Could you check a few things on this model? Use its own coordinates, in mm. A direction names the side the tool comes from. Round coordinates to 2 decimals unless told otherwise and drop trailing zeros. Loops run counter-clockwise (first coordinate to the right, second up) from the corner with the lowest first, then second, coordinate; pieces in that order, holes last. Notation, with made-up numbers: M -32.5,67 L -27.5,67 A12 cw -27.5,72 Z; hole C 50.5,84.5 d9. An arc over 180 degrees is marked long. One line per item, written item: value. Start each with the question number.
Q1. I'm going to push flat-ended pins straight in: pin 1 Ø1.4 at (x, y) = (77, 71) entering from +Z; pin 2 Ø5 at (x, y) = (55.12, 44.7) entering from +Z; pin 3 Ø2 at (y, z) = (64.5, 21) entering from -X. Where does each tip first touch, or does it pass through?
Q2. Imagine slicing it at A-A (y = 31.75). Please give me the cut outline in (x, z) (3 decimals).
Q3. Please list where these lines run through material, in increasing order: line 1 along Y through (x, z) = (5.08, 25.5) (3 decimals); line 2 along X through (y, z) = (78.5, 40); line 3 along Y through (x, z) = (7, 38.5).
Q4. Imagine slicing it at C-C (x = 67). Please give me the cut outline in (y, z), then the cut area to 3 significant figures.
Q5. Which directions (+Z, -Z, +X, -X, +Y, -Y) give clear straight access to the entire face, cutting with the end or side of a thin tool? Please do faces 1 (the face through (139.6, 93.2, 23.93)), 2 (the face through (14.41, 74.89, 10.71)), 3 (the face through (0, 60, 28)).
Q6. Thinking about a two-plate mould opening in Y: for faces 4 (the face through (13, 45, 5.08)), 5 (the face through (70, 121.412, 28)), 6 (the face through (141.478, 60, 28)), which applies, released by +Y, released by -Y, zero draft, split by the parting line, or undercut?
Q7. Imagine slicing it at B-B (z = 52.5). Give the number of separate pieces and of enclosed holes in the cut face, then the cut area to 3 significant figures.
from build123d import *

# Parameters (mm, degrees)
SKETCH1_W           = 141.478
SKETCH1_H           = 121.412
BOSS_EXTRUDE1_DEPTH = 5.08
SKETCH2_W           = 141.478
SKETCH2_H           = 121.412
SKETCH2_W_2         = 133.858
SKETCH2_H_2         = 113.792
BOSS_EXTRUDE2_DEPTH = 50.8
SKETCH3_W           = 10.16
SKETCH3_H           = 10.16
SKETCH3_R           = 1.397
BOSS_EXTRUDE3_DEPTH = 50.8
SKETCH4_R           = 9.525
CUT_EXTRUDE1_DEPTH  = 50.8
SKETCH5_R           = 3.175
CUT_EXTRUDE2_DEPTH  = 50.8
SKETCH6_R           = 5.352500138
SKETCH6_R_2         = 1.742129358
SKETCH6_R_3         = 4.222417447
SKETCH6_R_4         = 1.7145
SKETCH6_R_5         = 4.579780215
SKETCH6_R_6         = 1.684043279
SKETCH6_R_7         = 3.988290748
SKETCH6_R_8         = 1.731852199
SKETCH6_R_9         = 4.015615957
SKETCH6_R_10        = 1.588571248
SKETCH6_R_11        = 3.768246572
SKETCH6_R_12        = 1.460999264
SKETCH6_R_13        = 2.921
SKETCH6_R_14        = 1.397
SKETCH6_R_15        = 2.54
BOSS_EXTRUDE4_DEPTH = 11.43


with BuildPart() as part:
    # Sketch1 → Boss-Extrude1 (new body)
    with BuildSketch(Plane.XY):
        with Locations((70.739, 60.706)):
            Rectangle(SKETCH1_W, SKETCH1_H)
    extrude(amount=BOSS_EXTRUDE1_DEPTH)

    # Sketch2 → Boss-Extrude2 (add)
    with BuildSketch(Plane.XY.offset(5.08)):
        with Locations((70.739, 60.706)):
            Rectangle(SKETCH2_W, SKETCH2_H)
        with Locations((70.739, 60.706)):
            Rectangle(SKETCH2_W_2, SKETCH2_H_2, mode=Mode.SUBTRACT)
    extrude(amount=BOSS_EXTRUDE2_DEPTH)

    # Sketch3 → Boss-Extrude3 (add)
    # profile 1 of 4: a face of its own
    with BuildSketch(Plane.XY.offset(5.08)):
        with Locations((5.08, 116.332)):
            Rectangle(SKETCH3_W, SKETCH3_H)
        with Locations((5.08, 116.332)):
            Circle(SKETCH3_R, mode=Mode.SUBTRACT)
    # profile 2 of 4: a face of its own
    with BuildSketch(Plane.XY.offset(5.08)):
        with Locations((5.08, 5.08)):
            Rectangle(SKETCH3_W, SKETCH3_H)
        with Locations((5.08, 5.08)):
            Circle(SKETCH3_R, mode=Mode.SUBTRACT)
    # profile 3 of 4: a face of its own
    with BuildSketch(Plane.XY.offset(5.08)):
        with Locations((136.398, 5.08)):
            Rectangle(SKETCH3_W, SKETCH3_H)
        with Locations((136.398, 5.08)):
            Circle(SKETCH3_R, mode=Mode.SUBTRACT)
    # profile 4 of 4: a face of its own
    with BuildSketch(Plane.XY.offset(5.08)):
        with Locations((136.398, 116.332)):
            Rectangle(SKETCH3_W, SKETCH3_H)
        with Locations((136.398, 116.332)):
            Circle(SKETCH3_R, mode=Mode.SUBTRACT)
    extrude(amount=BOSS_EXTRUDE3_DEPTH)

    # Sketch4 → Cut-Extrude1 (cut)
    with BuildSketch(Plane(origin=(141.478, 0, 0), x_dir=(0, 0, -1), z_dir=(1, 0, 0))):
        with Locations((-25.4, 31.75)):
            Circle(SKETCH4_R)
    extrude(amount=-CUT_EXTRUDE1_DEPTH, mode=Mode.SUBTRACT)

    # Sketch5 → Cut-Extrude2 (cut)
    with BuildSketch(Plane(origin=(141.478, 0, 0), x_dir=(0, 0, -1), z_dir=(1, 0, 0))):
        with Locations((-25.4, 96.012)):
            Circle(SKETCH5_R)
    extrude(amount=-CUT_EXTRUDE2_DEPTH, mode=Mode.SUBTRACT)

    # Sketch6 → Boss-Extrude4 (add)
    # profile 1 of 9: a face of its own
    with BuildSketch(Plane.XY.offset(5.08)):
        with Locations(Location((56.555179335, 108.156736707, 0), (0, 0, 180))):
            Circle(SKETCH6_R)
        with Locations((56.555179335, 108.156736707)):
            Circle(SKETCH6_R_2, mode=Mode.SUBTRACT)
    # profile 2 of 9: a face of its own
    with BuildSketch(Plane.XY.offset(5.08)):
        with Locations(Location((56.555179335, 76.533736707, 0), (0, 0, 180))):
            Circle(SKETCH6_R_3)
        with Locations((56.555179335, 76.533736707)):
            Circle(SKETCH6_R_4, mode=Mode.SUBTRACT)
    # profile 3 of 9: a face of its own
    with BuildSketch(Plane.XY.offset(5.08)):
        with Locations(Location((14.772179335, 76.533736707, 0), (0, 0, 180))):
            Circle(SKETCH6_R_5)
        with Locations((14.772179335, 76.533736707)):
            Circle(SKETCH6_R_6, mode=Mode.SUBTRACT)
    # profile 4 of 9: a face of its own
    with BuildSketch(Plane.XY.offset(5.08)):
        with Locations(Location((14.772179335, 108.156736707, 0), (0, 0, 180))):
            Circle(SKETCH6_R_7)
        with Locations((14.772179335, 108.156736707)):
            Circle(SKETCH6_R_8, mode=Mode.SUBTRACT)
    # profile 5 of 9: a face of its own
    with BuildSketch(Plane.XY.offset(5.08)):
        with Locations(Location((55.116978912, 44.699028107, 0), (0, 0, 180))):
            Circle(SKETCH6_R_9)
        with Locations((55.116978912, 44.699028107)):
            Circle(SKETCH6_R_10, mode=Mode.SUBTRACT)
    # profile 6 of 9: a face of its own
    with BuildSketch(Plane.XY.offset(5.08)):
        with Locations(Location((12.825978912, 44.699028107, 0), (0, 0, 180))):
            Circle(SKETCH6_R_11)
        with Locations((12.825978912, 44.699028107)):
            Circle(SKETCH6_R_12, mode=Mode.SUBTRACT)
    # profile 7 of 9: a face of its own
    with BuildSketch(Plane.XY.offset(5.08)):
        with Locations(Location((114.503593068, 107.959774234, 0), (0, 0, 180))):
            Circle(SKETCH6_R_13)
        with Locations((114.503593068, 107.959774234)):
            Circle(SKETCH6_R_14, mode=Mode.SUBTRACT)
    # profile 8 of 9: a face of its own
    with BuildSketch(Plane.XY.offset(5.08)):
        with Locations(Location((76.911593068, 71.129774234, 0), (0, 0, 180))):
            Circle(SKETCH6_R_15)
        with Locations((76.911593068, 71.129774234)):
            Circle(SKETCH6_R_14, mode=Mode.SUBTRACT)
    # profile 9 of 9: a face of its own
    with BuildSketch(Plane.XY.offset(5.08)):
        with Locations(Location((77.673593068, 107.959774234, 0), (0, 0, 180))):
            Circle(SKETCH6_R_13)
        with Locations((77.673593068, 107.959774234)):
            Circle(SKETCH6_R_14, mode=Mode.SUBTRACT)
    extrude(amount=BOSS_EXTRUDE4_DEPTH)


solid = part.part
Report:
1. pin 1: stops at z = 5.08
1. pin 2: stops at z = 16.51
1. pin 3: stops at x = 0
2. outline: M 0,0 L 141.478,0 L 141.478,15.875 L 137.668,15.875 L 137.668,5.08 L 3.81,5.08 L 3.81,55.88 L 0,55.88 Z; M 137.668,34.925 L 141.478,34.925 L 141.478,55.88 L 137.668,55.88 Z
3. line 1: y = 0 to 3.81, 6.477 to 10.16, 111.252 to 114.935, 117.602 to 121.412
3. line 2: x = 0 to 3.81, 137.67 to 141.48
3. line 3: y = 0 to 10.16, 111.25 to 121.41
4. outline: M 0,0 L 121.41,0 L 121.41,55.88 L 117.6,55.88 L 117.6,5.08 L 3.81,5.08 L 3.81,55.88 L 0,55.88 Z
4. area: 1,000 mm²
5. face 1: +X
5. face 2: +Z
5. face 3: +Z, -Z, -X, +Y, -Y
6. face 4: undercut
6. face 5: released by +Y
6. face 6: zero draft
7. separate pieces: 1
7. enclosed holes: 5
7. area: 2,080 mm²
